from build123d import *

# Parameters (mm, degrees)
BOSS_EXTRUDE1_DEPTH                               = 7
CSK_FOR_0_FLAT_HEAD_MACHINE_SCREW_100_D           = 1.778
CSK_FOR_0_FLAT_HEAD_MACHINE_SCREW_100_CSINK_D     = 3.0226
CSK_FOR_0_FLAT_HEAD_MACHINE_SCREW_100_CSINK_ANGLE = 100


with BuildPart() as part:
    # Sketch1 → Boss-Extrude1 (new body)
    with BuildSketch(Plane(origin=(0, 0, 0), x_dir=(1, 0, 0), z_dir=(0, 1, 0))):
        with BuildLine():
            Line((-7.26, 0), (-3.26, 0))
            ThreePointArc((-3.26, 0), (0, -3.26), (3.26, 0))
            Line((3.26, 0), (7.26, 0))
            Line((7.26, 0), (7.26, -5))
            Line((7.26, -5), (-7.26, -5))
            Line((-7.26, -5), (-7.26, 0))
        make_face()
    extrude(amount=BOSS_EXTRUDE1_DEPTH)

    # CSK for #0 Flat Head Machine Screw (100)1 (through all)
    with Locations(Plane.XY.offset(5)):
        with Locations((-5.26, 3.5), (5.26, 3.5)):
            CounterSinkHole(CSK_FOR_0_FLAT_HEAD_MACHINE_SCREW_100_D / 2, CSK_FOR_0_FLAT_HEAD_MACHINE_SCREW_100_CSINK_D / 2, counter_sink_angle=CSK_FOR_0_FLAT_HEAD_MACHINE_SCREW_100_CSINK_ANGLE)


solid = part.part
Read the model definition and answer for the solid it produces. Units are mm, in the model's axes. Give positions to 0.01 mm unless a question says otherwise; leave off trailing zeros. Write each loop counter-clockwise with the first axis right and the second up, starting at its lowest first coordinate (ties: lowest second). Pieces come first, ordered by that corner, then holes. Notation, with made-up numbers: (59.25, 54.25) - (79.25, 54.25) arc R18 cw to (79.25, 58.25) - close; hole circle Ø1 at (-3, -35). An arc over 180 degrees is marked (long way). Use CSV: the item, a comma, the result in double quotes. Start each with the question number.
(1) Find section B-B (z = 2.5). Give the vertices of the cut face in (x, y), plus the area to 3 significant figures.
(2) Determine the mould class of faces 1 (the flat face through (-7.26, 3, 3)), 2 (the flat face through (0, 0, 4)), 3 (the flat face through (0, 7, 4)), 4 (the cylindrical face through (4.412, 3.767, 2.208)) for opening direction Y: +Y half, -Y half, draft (parallel to the pull), parting line (faces both ways), or undercut.
(3) Find section A-A (x = 5.26). Give the vertices of the cut face in (y, z).
(4) Consider line 1 along X through (y, z) = (3.5, 2.6); line 2 along Y through (x, z) = (5.26, 1.6); line 3 along X through (y, z) = (3.5, 1.8). Determine where each line is inside the solid, lowest interval first.
(5) Find section C-C (y = 6). Give the vertices of the cut face in (x, z).
(6) Find section D-D (z = 3.65). Give the vertices of the cut face in (x, y).
Findings below:
1,outline,"(-7.26, 0) - (-2.09, 0) - (-2.09, 7) - (-7.26, 7) - close; (2.09, 0) - (7.26, 0) - (7.26, 7) - (2.09, 7) - close; hole circle Ø1.78 at (-5.26, 3.5); hole circle Ø1.78 at (5.26, 3.5)"
1,area,"67.4 mm2"
2,face 1,"draft"
2,face 2,"-Y half"
2,face 3,"+Y half"
2,face 4,"undercut"
3,outline,"(0, 0) - (2.61, 0) - (2.61, 4.48) - (1.99, 5) - (0, 5) - close; (4.39, 0) - (7, 0) - (7, 5) - (5.01, 5) - (4.39, 4.48) - close"
4,line 1,"-7.26 to -6.15, -4.37 to -1.97, 1.97 to 4.37, 6.15 to 7.26"
4,line 2,"0 to 2.61, 4.39 to 7"
4,line 3,"-7.26 to -6.15, -4.37 to -2.72, 2.72 to 4.37, 6.15 to 7.26"
5,outline,"(-7.26, 0) - (-3.26, 0) arc R3.26 cw to (3.26, 0) - (7.26, 0) - (7.26, 5) - (-7.26, 5) - close"
6,outline,"(-7.26, 0) - (7.26, 0) - (7.26, 7) - (-7.26, 7) - close; hole circle Ø1.78 at (-5.26, 3.5); hole circle Ø1.78 at (5.26, 3.5)"
